from build123d import *

# Parameters (mm, degrees)
F1_DEPTH = 8
F3_D     = 6.6


with BuildPart() as f1:
    # F0 (on Top) → F1 (new body)
    with BuildSketch(Plane.XY):
        with BuildLine():
            ThreePointArc((-24.494897, -25), (-35, 0), (-24.494897, 25))
            ThreePointArc((-24.494897, 25), (-23.106602, 26.288495), (-21.650635, 27.5))
            Line((-21.650635, 27.5), (-44.650635, 27.5))
            Line((-44.650635, 27.5), (-44.650635, -27.5))
            Line((-44.650635, -27.5), (-21.650635, -27.5))
            ThreePointArc((-21.650635, -27.5), (-23.106602, -26.288495), (-24.494897, -25))
        make_face()
    extrude(amount=F1_DEPTH)

    # F3 (through all)
    with Locations(Plane(origin=(0, 0, 0), x_dir=(1, 0, 0), z_dir=(0, 0, -1))):
        with Locations((-36.650635, 20), (-36.650635, -20)):
            Hole(F3_D / 2)


solid = f1.part
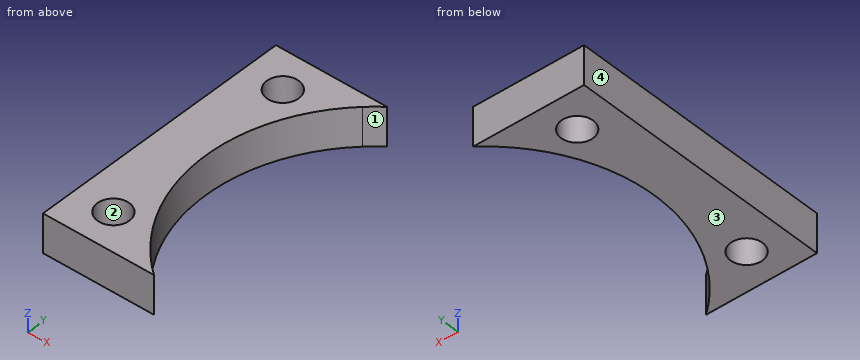
Work out the finished part from the listing and answer in its coordinate system (mm). Face numbers are marked on the shaded views. Round coordinates to 2 decimals unless told otherwise and drop trailing zeros. Write each loop counter-clockwise with the first axis right and the second up, starting at its lowest first coordinate (ties: lowest second). Pieces come first, ordered by that corner, then holes.
1) The mould has two halves that part along X. Classify the marked faces 1, 2, 3 and 4: pulls with the +X half, pulls with the -X half, needs draft (parallel to the pull), parting line crosses it, or undercut.
2) Straight lines are drawn through the part: line 1 (Y direction, x = -38.25, z = 2); line 2 (Y direction, x = -35.25, z = 0.75); line 3 (X direction, y = -20, z = 4.75). For each, find the intervals that lie inside material, in ascending order.
3) A cutting plane is placed at D-D (x = -38.5). Give the vertices of the cut face in (y, z).
4) A cutting plane is placed at A-A (x = -28.5). Give the vertices of the cut face in (y, z), plus the area to 3 significant figures.
5) Given pin 1 Ø3 at (y, z) = (8.5, 3) entering from +X, flat-ended and moving along its own axis, determine where the tip first touches the part or whether it passes through.
6) A cutting plane is placed at B-B (z = 5.5). Give the vertices of the cut face in (x, y).
7) A cutting plane is placed at C-C (y = 22.5). Give the vertices of the cut face in (x, z), plus the area to 3 significant figures.
Completed:
1. face 1: pulls with the +X half
1. face 2: undercut
1. face 3: needs draft
1. face 4: pulls with the -X half
2. line 1: y = -27.5 to -22.89, -17.11 to 17.11, 22.89 to 27.5
2. line 2: y = -27.5 to -22.99, -17.01 to 17.01, 22.99 to 27.5
2. line 3: x = -44.65 to -39.95, -33.35 to -28.72
3. outline: (-27.5, 0) - (-22.73, 0) - (-22.73, 8) - (-27.5, 8) - close; (-17.27, 0) - (17.27, 0) - (17.27, 8) - (-17.27, 8) - close; (22.73, 0) - (27.5, 0) - (27.5, 8) - (22.73, 8) - close
4. outline: (-27.5, 0) - (-20.32, 0) - (-20.32, 8) - (-27.5, 8) - close; (20.32, 0) - (27.5, 0) - (27.5, 8) - (20.32, 8) - close
4. area: 115 mm2
5. pin 1: stops at x = -33.54
6. outline: (-44.65, -27.5) - (-21.65, -27.5) arc R35 cw to (-24.49, -25) arc R35 cw to (-24.49, 25) arc R35 cw to (-21.65, 27.5) - (-44.65, 27.5) - close; hole circle Ø6.6 at (-36.65, -20); hole circle Ø6.6 at (-36.65, 20)
7. outline: (-44.65, 0) - (-38.8, 0) - (-38.8, 8) - (-44.65, 8) - close; (-34.5, 0) - (-26.81, 0) - (-26.81, 8) - (-34.5, 8) - close
7. area: 108 mm2
